Design review of the part built by this model. Coordinates are the model's own, in mm. Face numbers are marked on the shaded views. A direction names the side the tool comes from. Give positions to 0.01 mm unless a question says otherwise; leave off trailing zeros. Loops run counter-clockwise (first coordinate to the right, second up) from the corner with the lowest first, then second, coordinate; pieces in that order, holes last. Notation, with made-up numbers: M 67,76.5 L 86,76.5 A27 ccw 86,110.5 Z; hole C 49.25,56.25 d11. An arc over 180 degrees is marked long. Use a Markdown table: item, result. Add a question column.
(1) For the marked faces 1, 2, 3 and 4, list the 3-axis set-ups (+Z, -Z, +X, -X, +Y, -Y) from which the entire face can be reached by the end or side of a thin tool; tool diameter is ignored.
(2) Add section B-B, the plane z = 25. Give the boundary of the cut face in (x, y).
(3) For probe 1 along Y at (x, z) = (5, 16); probe 2 along Y at (x, z) = (42.5, 19.15); probe 3 along X at (y, z) = (-28.5, 11), list the stretches that pass through material, from the lowest coordinate up.
(4) Draft analysis for pull direction Y (two halves, no side actions). For the marked faces 5, 6 and 7, state which applies: pulls with the +Y half, pulls with the -Y half, needs draft (parallel to the pull), parting line crosses it, or undercut.
(5) Add section C-C, the plane y = -4.5. State how many separate pieces and enclosed holes the cut face has, then the cut area to 3 significant figures.
(6) Add section D-D, the plane x = 42.5. Give the boundary of the cut face in (y, z).
(7) Insertion check: pin 1 Ø2.5 at (x, z) = (58, 24.5) entering from -Y; pin 2 Ø8 at (x, y) = (112.5, -4.5) entering from +Z; pin 3 Ø5 at (x, z) = (3.5, 7) entering from +Y. Each pin has a flat end and moves straight along its axis. Give the tip position at first contact, or say it passes through.
(8) Add section A-A, the plane x = 60. Give the boundary of the cut face in (y, z).
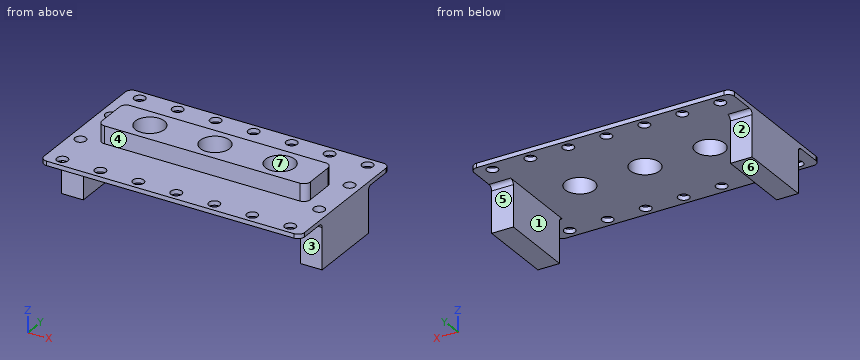
```python
from build123d import *

# Parameters (mm, degrees)
F0_W      = 120
F0_H      = 67.5
F1_DEPTH  = 20
F2_W      = 96
F2_H      = 19.5
F3_DEPTH  = 8
F4_R      = 6.75
F5_DEPTH  = 25
F7_DEPTH  = 18
F8_R      = 2.55
F9_DEPTH  = 25
F10_R     = 3
F11_R     = 3
F12_W     = 10
F12_H     = 35
F13_DEPTH = 3
F14_R     = 2
F15_R     = 2.55
F16_DEPTH = 10


with BuildPart() as f1:
    # F0 (on Top) → F1 (new body)
    with BuildSketch(Plane.XY):
        with Locations((60, -33.75)):
            Rectangle(F0_W, F0_H)
    extrude(amount=F1_DEPTH)

    # F2 (on face) → F3 (join)
    with BuildSketch(Plane.XY.offset(20)):
        with Locations((60, -33.75)):
            Rectangle(F2_W, F2_H)
    extrude(amount=F3_DEPTH)

    # F4 (on face) → F5 (cut)
    with BuildSketch(Plane.XY.offset(28)):
        with Locations((60, -33.75)):
            Circle(F4_R)
        with Locations((30, -33.75)):
            Circle(F4_R)
        with Locations((90, -33.75)):
            Circle(F4_R)
    extrude(amount=-F5_DEPTH, mode=Mode.SUBTRACT)

    # F6 (on face) → F7 (cut)
    with BuildSketch(Plane(origin=(0, 0, 0), x_dir=(1, 0, 0), z_dir=(0, 0, -1))):
        Polygon((10, 0), (110, 0), (120, 0), (120, 16.25), (110, 16.25), (110, 51.25), (120, 51.25), (120, 67.5), (110, 67.5), (10, 67.5), (0, 67.5), (0, 51.25), (10, 51.25), (10, 16.25), (0, 16.25), (0, 0), align=None)
    extrude(amount=-F7_DEPTH, mode=Mode.SUBTRACT)

    # F8 (on face) → F9 (cut)
    with BuildSketch(Plane.XY.offset(20)):
        with Locations((7.5, -4.5)):
            Circle(F8_R)
        with Locations((7.5, -63)):
            Circle(F8_R)
        with Locations((25, -4.5)):
            Circle(F8_R)
        with Locations((25, -63)):
            Circle(F8_R)
        with Locations((42.5, -4.5)):
            Circle(F8_R)
        with Locations((42.5, -63)):
            Circle(F8_R)
        with Locations((60, -4.5)):
            Circle(F8_R)
        with Locations((60, -63)):
            Circle(F8_R)
        with Locations((77.5, -4.5)):
            Circle(F8_R)
        with Locations((77.5, -63)):
            Circle(F8_R)
        with Locations((95, -4.5)):
            Circle(F8_R)
        with Locations((95, -63)):
            Circle(F8_R)
        with Locations((112.5, -4.5)):
            Circle(F8_R)
        with Locations((112.5, -63)):
            Circle(F8_R)
    extrude(amount=-F9_DEPTH, mode=Mode.SUBTRACT)

    # F10
    f10_edges = [f1.edges().sort_by_distance(p)[0] for p in [
        (108, -43.5, 24),
        (108, -24, 24),
        (12, -24, 24),
        (12, -43.5, 24),
    ]]
    fillet(f10_edges, radius=F10_R)

    # F11
    f11_edges = [f1.edges().sort_by_distance(p)[0] for p in [
        (120, 0, 19),
        (120, -67.5, 19),
        (0, 0, 19),
        (0, -67.5, 19),
    ]]
    fillet(f11_edges, radius=F11_R)

    # F12 (on face) → F13 (join)
    with BuildSketch(Plane(origin=(0, 0, 0), x_dir=(1, 0, 0), z_dir=(0, 0, -1))):
        with Locations((115, 33.75)):
            Rectangle(F12_W, F12_H)
        with Locations((5, 33.75)):
            Rectangle(F12_W, F12_H)
    extrude(amount=F13_DEPTH)

    # F14
    f14_edges = [f1.edges().sort_by_distance(p)[0] for p in [
        (115, -51.25, 18),
        (115, -16.25, 18),
        (5, -16.25, 18),
        (5, -51.25, 18),
    ]]
    fillet(f14_edges, radius=F14_R)

    # F15 (on face) → F16 (cut)
    with BuildSketch(Plane.XY.offset(20)):
        with Locations((115, -22.25)):
            Circle(F15_R)
        with Locations((115, -45.25)):
            Circle(F15_R)
        with Locations((5, -45.25)):
            Circle(F15_R)
        with Locations((5, -22.25)):
            Circle(F15_R)
    extrude(amount=-F16_DEPTH, mode=Mode.SUBTRACT)


solid = f1.part
```
Established:
| question | item | result |
|---|---|---|
| 1 | face 1 | -Z, +Y, -Y |
| 1 | face 2 | -Z, +X, -X, +Y |
| 1 | face 3 | -Z, +X, -X, -Y |
| 1 | face 4 | +Z, +X, -X, -Y |
| 2 | outline | M 12,-40.5 A3 ccw 15,-43.5 L 105,-43.5 A3 ccw 108,-40.5 L 108,-27 A3 ccw 105,-24 L 15,-24 A3 ccw 12,-27 Z; hole C 30,-33.75 d13.5; hole C 60,-33.75 d13.5; hole C 90,-33.75 d13.5 |
| 3 | probe 1 | -51.25 to -47.8, -42.7 to -24.8, -19.7 to -16.25 |
| 3 | probe 2 | -67.5 to -65.55, -60.45 to -7.05, -1.95 to 0 |
| 3 | probe 3 | 0 to 10, 110 to 120 |
| 4 | face 5 | pulls with the +Y half |
| 4 | face 6 | needs draft |
| 4 | face 7 | undercut |
| 5 | separate pieces | 8 |
| 5 | enclosed holes | 0 |
| 5 | area | 169 mm^2 |
| 6 | outline | M -67.5,18 L -65.55,18 L -65.55,20 L -67.5,20 Z; M -60.45,18 L -7.05,18 L -7.05,20 L -24,20 L -24,28 L -43.5,28 L -43.5,20 L -60.45,20 Z; M -1.95,18 L 0,18 L 0,20 L -1.95,20 Z |
| 7 | pin 1 | y = -43.5 |
| 7 | pin 2 | z = 20 |
| 7 | pin 3 | y = -16.25 |
| 8 | outline | M -67.5,18 L -65.55,18 L -65.55,20 L -67.5,20 Z; M -60.45,18 L -40.5,18 L -40.5,28 L -43.5,28 L -43.5,20 L -60.45,20 Z; M -27,18 L -7.05,18 L -7.05,20 L -24,20 L -24,28 L -27,28 Z; M -1.95,18 L 0,18 L 0,20 L -1.95,20 Z |
